Input: part model. Units: mm. Frame: model coordinates. A direction names the side the tool comes from. Give positions to 0.01 mm unless a question says otherwise; leave off trailing zeros. Loops run counter-clockwise (first coordinate to the right, second up) from the corner with the lowest first, then second, coordinate; pieces in that order, holes last. Notation, with made-up numbers: M -33.5,-34 L -14.5,-34 A4 ccw -14.5,-30 Z; hole C 40,-26.75 d4. An arc over 180 degrees is marked long. Answer as a JSON object with one key per item and string values. Group by question number.
```python
from build123d import *

# Parameters (mm, degrees)
SKETCH1_R           = 7.5
SKETCH1_R_2         = 5
BOSS_EXTRUDE1_DEPTH = 5
SKETCH2_W           = 30
SKETCH2_H           = 30
BOSS_EXTRUDE2_DEPTH = 2.5
FILLET1_R           = 5
FILLET2_R           = 1.3


with BuildPart() as part:
    # Sketch1 → Boss-Extrude1 (new body)
    with BuildSketch(Plane.XY):
        Circle(SKETCH1_R)
        Circle(SKETCH1_R_2, mode=Mode.SUBTRACT)
    extrude(amount=BOSS_EXTRUDE1_DEPTH)

    # Sketch2 → Boss-Extrude2 (add)
    with BuildSketch(Plane.XY.offset(5)):
        Rectangle(SKETCH2_W, SKETCH2_H)
    extrude(amount=BOSS_EXTRUDE2_DEPTH)

    # Fillet1
    fillet1_edges = [part.edges().sort_by_distance(p)[0] for p in [
        (15, -15, 6.25),
        (15, 15, 6.25),
        (-15, 15, 6.25),
        (-15, -15, 6.25),
    ]]
    fillet(fillet1_edges, radius=FILLET1_R)

    # Fillet2
    fillet2_edges = [part.edges().sort_by_distance(p)[0] for p in [
        (-7.5, 0, 5),
    ]]
    fillet(fillet2_edges, radius=FILLET2_R)


solid = part.part
```
1. Reachability of faces 4 (the cylindrical face through (13, 14, 6)), 5 (the flat face through (0, 0, 5)) from +Z, -Z, +X, -X, +Y, -Y: full face, straight path, thin tool, end or side. Return the list, or none.
2. First-contact query: P1, Ø1, axis at x = 11, z = 5.5, coming from the -Y side; P2, Ø2, axis at y = -0.5, z = 3, coming from the +X side; P3, Ø3, axis at x = 2, y = 2, coming from the -Z side. Flat tips, straight axial feed; report the tip coordinate or a pass-through.
3. Section D-D (z = 1.75). Output: boundary loops of the cut face in (x, y).
4. Material intervals for L1, parallel to Y at x = 0, z = 2.3; L2, parallel to Z at x = -4.25, y = -8.75; L3, parallel to Y at x = -1.5, z = 2.5, sorted ascending.
5. Mould query, pull axis X, two halves, no side actions, for faces 1 (the cylindrical face through (-1.08, -4.88, 2.46)), 2 (the flat face through (0, 0, 7.5)), 3 (the flat face through (-15, 0, 6)). Classes: pulls with the +X half, pulls with the -X half, needs draft (parallel to the pull), parting line crosses it, or undercut.
6. Section B-B (x = 0). Output: boundary loops of the cut face in (y, z).
7. Section A-A (z = 6.75). Output: boundary loops of the cut face in (x, y).
Geometry results:
{
 "1": {"face 4": "+Z, -Z, +X, +Y", "face 5": "-Z"},
 "2": {"P1": "y = -14.97", "P2": "x = 7.52", "P3": "z = 5"},
 "3": {"outline": "C 0,0 d15; hole C 0,0 d10"},
 "4": {"L1": "-7.5 to -5, 5 to 7.5", "L2": "5 to 7.5", "L3": "-7.35 to -4.77, 4.77 to 7.35"},
 "5": {"face 1": "undercut", "face 2": "needs draft", "face 3": "pulls with the -X half"},
 "6": {"outline": "M -15,5 L -8.8,5 A1.3 cw -7.5,3.7 L -7.5,0 L -5,0 L -5,5 L 5,5 L 5,0 L 7.5,0 L 7.5,3.7 A1.3 cw 8.8,5 L 15,5 L 15,7.5 L -15,7.5 Z"},
 "7": {"outline": "M -15,-10 A5 ccw -10,-15 L 10,-15 A5 ccw 15,-10 L 15,10 A5 ccw 10,15 L -10,15 A5 ccw -15,10 Z"}
}
